from build123d import *

# Parameters (mm, degrees)
EXTRUDE_1_DEPTH = 10


with BuildPart() as part:
    # Эскиз1 → Бобышка-Вытянуть1 (new body)
    with BuildSketch(Plane(origin=(0, 0, 0), x_dir=(1, 0, 0), z_dir=(0, 1, 0))):
        with BuildLine():
            Line((-16.5, 0), (-16.5, -10))
            Line((-16.5, -10), (-13.124404748, -10))
            ThreePointArc((-13.124404748, -10), (0, -16.5), (13.124404748, -10))
            Line((13.124404748, -10), (16.5, -10))
            Line((16.5, -10), (16.5, 0))
            Line((16.5, 0), (26.5, 0))
            Line((26.5, 0), (26.5, 5))
            Line((26.5, 5), (11.5, 5))
            Line((11.5, 5), (11.5, 0))
            ThreePointArc((11.5, 0), (0, -11.5), (-11.5, 0))
            Line((-11.5, 0), (-11.5, 5))
            Line((-11.5, 5), (-26.5, 5))
            Line((-26.5, 5), (-26.5, 0))
            Line((-26.5, 0), (-16.5, 0))
        make_face()
    extrude(amount=EXTRUDE_1_DEPTH)


solid = part.part
The model under review builds one solid part; all positions refer to its coordinate system, in mm. A direction names the side the tool comes from. Give positions to 0.01 mm unless a question says otherwise; leave off trailing zeros. Loops run counter-clockwise (first coordinate to the right, second up) from the corner with the lowest first, then second, coordinate; pieces in that order, holes last. Notation, with made-up numbers: (70, -22.75) -> (83, -22.75) arc R19 ccw to (83, -14.75) -> close; hole circle Ø2 at (87, 0.5). An arc over 180 degrees is marked (long way). Put each result on its own line as item: value. Start each with the question number.
1. Wall thickness on probe 1 along X at (y, z) = (3.75, -3.25); probe 2 along X at (y, z) = (5, 0.5); probe 3 along Z at (x, y) = (-23, 8.75): over which ranges is each line inside the solid? List them lowest first.
2. We need section C-C on x = -15. State the section outline as (y, z) points.
3. Mouldability with a two-part tool opening along X and no side actions: class faces 5 (the face through (26.5, 5, -2)), 6 (the face through (0.253, 4.93, 11.497)), 7 (the face through (-15, 5, 10)), 8 (the face through (11.5, 5, -3)) as released by +X, released by -X, zero draft, split by the parting line, or undercut.
4. We need section B-B on y = 4.75. State the section outline as (x, z) points, then the cut area to 3 significant figures.
5. We need section A-A on z = -3.5. State the section outline as (x, y) points, then the cut area to 3 significant figures.
6. We need section D-D on z = 2.75. State the section outline as (x, y) points, then the cut area to 3 significant figures.
7. For faces 1 (the face through (-11.5, 5, -2)), 2 (the face through (15, 5, 10)), 3 (the face through (-16.5, 5, 5)), 4 (the face through (19, 5, -5)), list the 3-axis set-ups (+Z, -Z, +X, -X, +Y, -Y) from which the entire face can be reached by the end or side of a thin tool; tool diameter is ignored.
8. Clearance check with flat-ended pins moving along their axes: P1, Ø12, axis at x = -5.5, z = 9.5, coming from the -Y side; P2, Ø5, axis at y = 6, z = 5.5, coming from the +X side; P3, Ø1.7, axis at x = -14, y = 4, coming from the +Z side; P4, Ø2, axis at y = 3.5, z = 10.5, coming from the -X side. State where each tip first meets the part, or that it passes through.
Determined:
1. probe 1: -26.5 to -11.5, 11.5 to 26.5
1. probe 2: -16.5 to -11.49, 11.49 to 16.5
1. probe 3: -5 to 0
2. outline: (0, -5) -> (10, -5) -> (10, 10) -> (0, 10) -> close
3. face 5: released by +X
3. face 6: undercut
3. face 7: zero draft
3. face 8: undercut
4. outline: (-26.5, -5) -> (-11.5, -5) -> (-11.5, 0) arc R11.5 cw to (11.5, 0) -> (11.5, -5) -> (26.5, -5) -> (26.5, 0) -> (16.5, 0) -> (16.5, 10) -> (13.12, 10) arc R16.5 ccw to (-13.12, 10) -> (-16.5, 10) -> (-16.5, 0) -> (-26.5, 0) -> close
4. area: 391 mm^2
5. outline: (-26.5, 0) -> (-11.5, 0) -> (-11.5, 10) -> (-26.5, 10) -> close; (11.5, 0) -> (26.5, 0) -> (26.5, 10) -> (11.5, 10) -> close
5. area: 300 mm^2
6. outline: (-16.5, 0) -> (-11.17, 0) -> (-11.17, 10) -> (-16.5, 10) -> close; (11.17, 0) -> (16.5, 0) -> (16.5, 10) -> (11.17, 10) -> close
6. area: 107 mm^2
7. face 1: -Z, +Y, -Y
7. face 2: +Z, +X, +Y, -Y
7. face 3: +Z, -X, +Y, -Y
7. face 4: -Z, +X, -X, +Y, -Y
8. P1: y = 0
8. P2: x = 16.5
8. P3: z = 10
8. P4: x = -16.5
